from build123d import *

# Parameters (mm, degrees)
EXTRUDE_1_DEPTH          = 60
CUT_EXTRUDE_1_REACH      = 63.686
CUT_EXTRUDE_1_END_RADIUS = 40.2
SKETCH_2_R               = 3
CUT_EXTRUDE_2_DEPTH      = 3
FILLET_1_R               = 10


with BuildPart() as part:
    # Эскиз1 → Бобышка-Вытянуть1 (new body)
    with BuildSketch(Plane.XY):
        with BuildLine():
            Line((-12.5, -38.207198275), (-12.5, -33.207198275))
            Line((-12.5, -33.207198275), (12.5, -33.207198275))
            Line((12.5, -33.207198275), (12.5, -38.207198275))
            ThreePointArc((12.5, -38.207198275), (0, -40.2), (-12.5, -38.207198275))
        make_face()
    extrude(amount=EXTRUDE_1_DEPTH)

    # Вырез-Вытянуть1: up to this cylinder (the profile starts inside it)
    cut_extrude_1_end = Plane(origin=(0, 0, 30), z_dir=(0, 0, -1)) * Cylinder(CUT_EXTRUDE_1_END_RADIUS, 248.772, mode=Mode.PRIVATE)
    # Эскиз2 → Вырез-Вытянуть1 (cut, up to the surface)
    with BuildSketch(Plane(origin=(0, -33.207198275, 0), x_dir=(1, 0, 0), z_dir=(0, 1, 0)), mode=Mode.PRIVATE) as cut_extrude_1_sk1:
        with Locations(Location((0, -10, 0), (0, 0, 270))):
            Circle(SKETCH_2_R)
    cut_extrude_1_tool1 = extrude(cut_extrude_1_sk1.sketch, amount=-CUT_EXTRUDE_1_REACH, mode=Mode.PRIVATE) & cut_extrude_1_end
    add(cut_extrude_1_tool1.solids().sort_by_distance((0, -33.207198, 10))[0], mode=Mode.SUBTRACT)
    # Эскиз2 → Вырез-Вытянуть1 (cut, up to the surface)
    with BuildSketch(Plane(origin=(0, -33.207198275, 0), x_dir=(1, 0, 0), z_dir=(0, 1, 0)), mode=Mode.PRIVATE) as cut_extrude_1_sk2:
        with Locations(Location((0, -50, 0), (0, 0, 270))):
            Circle(SKETCH_2_R)
    cut_extrude_1_tool2 = extrude(cut_extrude_1_sk2.sketch, amount=-CUT_EXTRUDE_1_REACH, mode=Mode.PRIVATE) & cut_extrude_1_end
    add(cut_extrude_1_tool2.solids().sort_by_distance((0, -33.207198, 50))[0], mode=Mode.SUBTRACT)

    # Эскиз3 → Вырез-Вытянуть2 (cut)
    with BuildSketch(Plane(origin=(0, -33.207198275, 0), x_dir=(1, 0, 0), z_dir=(0, 1, 0))):
        Polygon((3.031088913, -4.75), (-3.031088913, -4.75), (-6.062177826, -10), (-3.031088913, -15.25), (3.031088913, -15.25), (6.062177826, -10), align=None)
        Polygon((3.031088913, -44.75), (-3.031088913, -44.75), (-6.062177826, -50), (-3.031088913, -55.25), (3.031088913, -55.25), (6.062177826, -50), align=None)
    extrude(amount=-CUT_EXTRUDE_2_DEPTH, mode=Mode.SUBTRACT)

    # Скругление1
    fillet_1_edges = [part.edges().sort_by_distance(p)[0] for p in [
        (-12.5, -35.707198275, 60),
        (-12.5, -35.707198275, 0),
        (12.5, -35.707198275, 0),
        (12.5, -35.707198275, 60),
    ]]
    fillet(fillet_1_edges, radius=FILLET_1_R)


solid = part.part
For this review, take the finished solid that the model builds, in its own axes (mm). A direction names the side the tool comes from. Round coordinates to 2 decimals unless told otherwise and drop trailing zeros. Order: outer loops, then holes, each group sorted by start corner. A loop starts at its lowest first (then second) coordinate and runs counter-clockwise, first axis right, second up. Notation, with made-up numbers: (-39.75, -35) -> (4.25, -35) arc R7 ccw to (4.25, -24) -> close; hole circle Ø1 at (16.5, 36). An arc over 180 degrees is marked (long way). Write item = value, one per line. Start each with the question number.
1) Tool access review of faces 1 (the face through (0, -38, 47)), 2 (the face through (4.568, -34.686, 47.412)): name each direction out of +Z, -Z, +X, -X, +Y, -Y from which nothing blocks a thin tool from reaching the whole face with its end or side.
2) The part is to be moulded in two halves that separate along Z. For faces 3 (the face through (9.49, -35.94, 2.85)), 4 (the face through (9.49, -35.94, 57.15)), 5 (the face through (0, -35, 4.75)), say which applies: +Z half, -Z half, draft (parallel to the pull), parting line (faces both ways), or undercut.
3) To check wall thickness, follow line 1 (Z direction, x = 0, y = -37.95); line 2 (Z direction, x = 1, y = -34); line 3 (X direction, y = -37.2, z = 10). State the ranges of each line that lie inside material, in increasing order. Write a range as from..to.
4) Take a section at C-C on z = 16.5. State the section outline as (x, y) points, plus the area to 3 significant figures.
5) Insertion check: pin 1 (10 mm diameter, centred on x = 0.5, z = 12.5, fed in from -Y); pin 2 (9.5 mm diameter, centred on x = 0, z = 10, fed in from +Y); pin 3 (1 mm diameter, centred on x = 5, y = -39.5, fed in from -Z); pin 4 (1 mm diameter, centred on x = 5, z = 41.5, fed in from -Y). Each pin has a flat end and moves straight along its axis. Give the tip position at first contact, or say it passes through.
6) Take a section at B-B on x = -5.5. State the section outline as (y, z) points, plus the area to 3 significant figures.
7) Take a section at D-D on z = 4. State the section outline as (x, y) points, plus the area to 3 significant figures.
8) Take a section at A-A on x = 0. State the section outline as (y, z) points, plus the area to 3 significant figures.
Verdict:
q1.face_1 = +Y, -Y
q1.face_2 = +Y
q2.face_3 = -Z half
q2.face_4 = +Z half
q2.face_5 = undercut
q3.line_1 = 0..7, 13..47, 53..60
q3.line_2 = 0..4.75, 15.25..44.75, 55.25..60
q3.line_3 = -12.5..-3, 3..12.5
q4.outline = (-12.5, -38.21) arc R40.2 ccw to (12.5, -38.21) -> (12.5, -33.21) -> (-12.5, -33.21) -> close
q4.area = 158 mm2
q5.pin_1 = -40.2
q5.pin_2 = -36.21
q5.pin_3 = 0.2
q5.pin_4 = -39.95
q6.outline = (-39.82, 0.46) -> (-33.21, 0.46) -> (-33.21, 9.03) -> (-36.21, 9.03) -> (-36.21, 10.97) -> (-33.21, 10.97) -> (-33.21, 49.03) -> (-36.21, 49.03) -> (-36.21, 50.97) -> (-33.21, 50.97) -> (-33.21, 59.54) -> (-39.82, 59.54) -> close
q6.area = 379 mm2
q7.outline = (-10.5, -38.8) arc R40.2 ccw to (10.5, -38.8) -> (10.5, -33.21) -> (-10.5, -33.21) -> close
q7.area = 137 mm2
q8.outline = (-40.2, 0) -> (-33.21, 0) -> (-33.21, 4.75) -> (-36.21, 4.75) -> (-36.21, 7) -> (-40.2, 7) -> close; (-40.2, 13) -> (-36.21, 13) -> (-36.21, 15.25) -> (-33.21, 15.25) -> (-33.21, 44.75) -> (-36.21, 44.75) -> (-36.21, 47) -> (-40.2, 47) -> close; (-40.2, 53) -> (-36.21, 53) -> (-36.21, 55.25) -> (-33.21, 55.25) -> (-33.21, 60) -> (-40.2, 60) -> close
q8.area = 309 mm2
